Geometry check sheet. Reference: the model listing, model coordinates, mm. A direction names the side the tool comes from. Coordinates: 2 decimals unless noted, no trailing zeros. Loops run counter-clockwise (first coordinate to the right, second up) from the corner with the lowest first, then second, coordinate; pieces in that order, holes last. Notation, with made-up numbers: M -1.5,28 L 18.5,28 A12 ccw 18.5,44 Z; hole C -40,22.5 d4. An arc over 180 degrees is marked long. Use CSV: the item, a comma, the result in double quotes.
Autodesk Inventor part; units mm, degrees
ref_plane "YZ Plane" through (0, 0, 0) normal (1, 0, 0) x (0, 1, 0)
ref_plane "XZ Plane" through (0, 0, 0) normal (0, 1, 0) x (-1, 0, 0)
ref_plane "XY Plane" through (0, 0, 0) normal (0, 0, 1) x (1, 0, 0)
sketch "Sketch1" plane through (0, 0, 0) normal (0, 0, 1) x (1, 0, 0)
  line L0 (350, -145) -> (-350, -145)
  line L1 (-350, -145) -> (-350, 145)
  line L2 (-350, 145) -> (350, 145)
  line L3 (350, 145) -> (350, -145)
  line L4 (350, -145) -> (-350, 145) construction
  line L5 (-350, -145) -> (350, 145) construction
  point P0 (0, 0)
  dimension "d0" = 290
  dimension "d1" = 700
extrude "Extrusion1" add sketch "Sketch1" along normal blind 3
sketch "Sketch2" plane through (0, 0, 3) normal (0, 0, 1) x (1, 0, 0)
  line L0 (-320, 115) -> (-155, 115)
  line L1 (-155, 115) -> (-155, -115)
  line L2 (-155, -115) -> (-320, -115)
  line L3 (-320, -115) -> (-320, 115)
  line L4 (-350, 145) -> (-350, -145)
  line L5 (350, 145) -> (-350, 145)
  line L6 (-350, -145) -> (350, -145)
  point P0 (0, 0)
  dimension "d4" = 30
  dimension "d5" = 30
  dimension "d6" = 30
  dimension "d7" = 165
extrude "Extrusion2" cut sketch "Sketch2" against normal blind 3
fillet "Fillet1" radius 30 4 edges at (-320, 115, 1.5) (-155, 115, 1.5) (-320, -115, 1.5) (-155, -115, 1.5)
mirror "Mirror1" about plane through (0, 0, 0) normal (1, 0, 0) of "Extrusion2", "Fillet1"
sketch "Sketch3" plane through (0, 0, 3) normal (0, 0, 1) x (1, 0, 0)
  line L0 (-290, 115) -> (-185, 115)
  line L1 (-155, 85) -> (-155, -85)
  line L2 (-185, -115) -> (-290, -115)
  line L3 (350, 145) -> (-350, 145)
  line L4 (-350, -145) -> (350, -145)
  line L5 (-350, 145) -> (-350, -145)
  line L6 (350, -145) -> (350, 145)
  line L7 (82.5, -115) -> (-82.5, -115)
  line L8 (-82.5, -115) -> (-82.5, 115)
  line L9 (-82.5, 115) -> (82.5, 115)
  line L10 (82.5, 115) -> (82.5, -115)
  line L11 (82.5, -115) -> (-82.5, 115) construction
  line L12 (-82.5, -115) -> (82.5, 115) construction
  line L13 (-320, -85) -> (-320, 85)
  point P0 (0, 0)
  dimension "d11" = 165
  dimension "d12" = 165
extrude "Extrusion3" cut sketch "Sketch3" against normal blind 3 contours L7 L8 L9 L10
fillet "Fillet2" radius 30 4 edges at (82.5, 115, 1.5) (-82.5, 115, 1.5) (-82.5, -115, 1.5) (82.5, -115, 1.5)
sketch "Sketch4" plane through (0, 0, 3) normal (0, 0, 1) x (1, 0, 0)
  line L0 (-350, 145) -> (-350, -145)
  line L1 (-350, -145) -> (350, -145)
  line L2 (-60, -145) -> (-50, -145)
  line L3 (-50, -145) -> (-50, -129.9972)
  line L4 (-50, -129.9972) -> (-60, -129.9972)
  line L5 (-60, -129.9972) -> (-60, -145)
  point P0 (0, 0)
  dimension "d16" = 290
  dimension "d17" = 10
extrude "Extrusion4" cut sketch "Sketch4" against normal blind 3
fillet "Fillet3" radius 5 2 edges at (-60, -129.9972, 1.5) (-50, -129.9972, 1.5)
mirror "Mirror2" about plane through (0, 0, 0) normal (1, 0, 0) of "Extrusion4", "Fillet3"
equation "\"d12\" = d11"
equation "\"d20\" = 0.5 * d17"
properties part number "GBX_020.1-front-MDF"
1. Section check D-D, the plane x = 173.5. Record the cut outline in (y, z).
The answers:
outline,"M -145,0 L -112.71,0 L -112.71,3 L -145,3 Z; M 112.71,0 L 145,0 L 145,3 L 112.71,3 Z"
2. Thickness scan on line 1 (X direction, y = 20.5, z = 2.65); line 2 (Y direction, x = 217.5, z = 1); line 3 (Y direction, x = -173, z = 0.15). Record the ranges inside material, lowest first. Write a range as [from, to].
The answers:
line 1,"[-350, -320], [-155, -82.5], [82.5, 155], [320, 350]"
line 2,"[-145, -115], [115, 145]"
line 3,"[-145, -112.5], [112.5, 145]"
3. Release check for a two-part mould opening along X. For faces 1 (the cylindrical face through (-163.555, -105.979, 1.479)), 2 (the cylindrical face through (-73.479, -106.445, 1.479)), 3 (the flat face through (-83, 2, 3)) record: +X half, -X half, draft (parallel to the pull), parting line (faces both ways), or undercut.
The answers:
face 1,"undercut"
face 2,"undercut"
face 3,"draft"
4. Section check A-A, the plane x = 257.5. Record the cut outline in (y, z).
The answers:
outline,"M -145,0 L -115,0 L -115,3 L -145,3 Z; M 115,0 L 145,0 L 145,3 L 115,3 Z"
5. Set-up check for faces 4 (the flat face through (-83, 2, 0)), 5 (the cylindrical face through (164.021, -106.445, 1.479)): record each of +Z, -Z, +X, -X, +Y, -Y from which the full face is reachable in a straight line by a thin tool's end or side.
The answers:
face 4,"-Z, +X, -X, +Y, -Y"
face 5,"+Z, -Z"
6. Section check C-C, the plane z = 2. Count the separate pieces of the cut face and the enclosed holes in it, plus the area to 3 significant figures.
The answers:
separate pieces,"1"
enclosed holes,"3"
area,"91,200 mm^2"
7. Section check B-B, the plane y = -55.5. Record the cut outline in (x, z).
The answers:
outline,"M -350,0 L -320,0 L -320,3 L -350,3 Z; M -155,0 L -82.5,0 L -82.5,3 L -155,3 Z; M 82.5,0 L 155,0 L 155,3 L 82.5,3 Z; M 320,0 L 350,0 L 350,3 L 320,3 Z"
